Source: CAD feature listing. Evaluate the final solid. Frame: model axes, mm. A direction names the side the tool comes from. Coordinates: 2 decimals unless noted, no trailing zeros. Order: outer loops, then holes, each group sorted by start corner. A loop starts at its lowest first (then second) coordinate and runs counter-clockwise, first axis right, second up. Notation, with made-up numbers: (-15.5, -9) - (34.5, -9) arc R17 ccw to (34.5, 15) - close; hole circle Ø7 at (-7.5, -11). An arc over 180 degrees is marked (long way). One line per question, with ' | ' between items. Start each with the question number.
(1) Access query for faces 1 (the flat face through (80, 2, 24.613)), 2 (the flat face through (61, 1.588, 35)), 3 (the flat face through (1.588, 1, 36)), 4 (the flat face through (61, 1.588, 5)). Directions: +Z, -Z, +X, -X, +Y, -Y. A direction counts if a zero-diameter tool reaches every point of the face in a straight line with its end or side. Return the directions, or none.
(2) Section C-C (x = 39). Return the cut outline in (y, z) (1 decimal).
(3) Section A-A (y = 2.65). Count the separate pieces of the cut face and the enclosed holes in it, then the cut area to 3 significant figures.
(4) Section B-B (x = 112). Return the cut outline in (y, z) (1 decimal), then the cut area to 3 significant figures.
(5) Draft query along X for faces 5 (the flat face through (63, 0, 19)), 6 (the flat face through (123.825, 2, 16)), 7 (the flat face through (106, 2, 14.77)), 8 (the flat face through (0, 2, 16)). Return one class per face: +X half, -X half, draft (parallel to the pull), parting line (faces both ways), or undercut.
(6) Contact query for flat-ended pins moving along their axis: P1, Ø1, axis at y = 2.5, z = 18, coming from the -X side; P2, Ø1.6, axis at y = 2, z = 35.5, coming from the -X side; P3, Ø1, axis at y = 1.5, z = 35, coming from the +X side. Output: stop coordinate, or through.
(7) Line query: line 1 along Z through (x, y) = (106.5, 3.05) (1 decimal); line 2 along Z through (x, y) = (43.5, 1.9) (1 decimal); line 3 along X through (y, z) = (0.8, 15) (1 decimal). Output: solid intervals per line, ascending.
Autodesk Inventor part; units mm, degrees
ref_plane "YZ Plane" through (0, 0, 0) normal (1, 0, 0) x (0, 1, 0)
ref_plane "XZ Plane" through (0, 0, 0) normal (0, 1, 0) x (-1, 0, 0)
ref_plane "XY Plane" through (0, 0, 0) normal (0, 0, 1) x (1, 0, 0)
sketch "Sketch1" plane through (0, 0, 0) normal (0, 1, 0) x (-1, 0, 0)
  line L0 (0, 0) -> (-123.825, 0)
  line L1 (-123.825, 0) -> (-123.825, 38.1)
  line L2 (-123.825, 38.1) -> (0, 38.1)
  line L3 (0, 38.1) -> (0, 0)
  dimension "d0" = 123.825
  dimension "d1" = 38.1
extrude "Extrusion1" add sketch "Sketch1" along normal blind 3.175
sketch "Sketch2" plane through (0, 3.175, 0) normal (0, 1, 0) x (1, 0, 0)
  line L0 (123.825, 0) -> (0, 0)
  line L1 (0, 0) -> (0, -38.1)
  line L2 (0, -38.1) -> (123.825, -38.1)
  line L3 (123.825, -38.1) -> (123.825, 0)
  line L4 (0, -36.5125) -> (123.825, -36.5125)
  line L5 (123.825, -36.5125) -> (123.825, -33.3121)
  line L6 (123.825, -33.3121) -> (0, -33.3121)
  line L7 (0, -33.3121) -> (0, -36.5125)
  line L8 (1.5875, -3.175) -> (122.2375, -3.175)
  line L9 (122.2375, -3.175) -> (122.2375, -6.604)
  line L10 (122.2375, -6.604) -> (1.5875, -6.604)
  line L11 (1.5875, -6.604) -> (1.5875, -3.175)
  dimension "d6" = 3.2004
  dimension "d7" = 1.5875
  dimension "d10" = 3.175
  dimension "d11" = 3.429
  dimension "d12" = 1.5875
  dimension "d13" = 1.5875
extrude "Extrusion2" cut sketch "Sketch2" against normal blind 1.5875 contours L3 L4 L1 L6
sketch "Sketch3" plane through (0, 3.175, 0) normal (0, 1, 0) x (1, 0, 0)
  line L0 (123.825, -33.3121) -> (123.825, 0)
  line L1 (123.825, 0) -> (0, 0)
  line L2 (0, 0) -> (0, -33.3121)
  line L3 (1.5875, -3.175) -> (122.2375, -3.175)
  line L4 (122.2375, -3.175) -> (122.2375, -6.604)
  line L5 (122.2375, -6.604) -> (1.5875, -6.604)
  line L6 (1.5875, -6.604) -> (1.5875, -3.175)
  dimension "d14" = 1.5875
  dimension "d15" = 1.5875
  dimension "d16" = 3.175
  dimension "d17" = 3.429
extrude "Extrusion3" cut sketch "Sketch3" against normal blind 1.5875
sketch "Sketch4" plane through (0, 3.175, 0) normal (0, 1, 0) x (1, 0, 0)
  line L0 (0, -38.1) -> (1.5875, -38.1)
  line L1 (1.5875, -38.1) -> (1.5875, -31.75)
  line L2 (1.5875, -31.75) -> (0, -31.75)
  line L3 (0, -31.75) -> (0, -38.1)
  line L4 (123.825, -38.1) -> (122.2375, -38.1)
  line L5 (122.2375, -38.1) -> (122.2375, -31.75)
  line L6 (122.2375, -31.75) -> (123.825, -31.75)
  line L7 (123.825, -31.75) -> (123.825, -38.1)
  point P0 (0, 0)
  dimension "d20" = 1.5875
  dimension "d21" = 6.35
  dimension "d22" = 6.35
  dimension "d23" = 1.5875
extrude "Extrusion4" cut sketch "Sketch4" against normal blind 25.4
fillet "Fillet1" radius 1.5875 1 edges at (122.2375, 1.5875, 31.75)
fillet "Fillet2" radius 1.5875 1 edges at (1.5875, 1.5875, 31.75)
sketch "Sketch5" plane through (0, 3.175, 0) normal (0, 1, 0) x (1, 0, 0)
  line L0 (1.5873, -33.3121) -> (122.2377, -33.3121)
  line L1 (74.9935, -21.0566) -> (84.1375, -21.0566)
  line L2 (84.1375, -21.0566) -> (84.1375, -24.6126)
  line L3 (84.1375, -24.6126) -> (74.9935, -24.6126)
  line L4 (74.9935, -24.6126) -> (74.9935, -21.0566)
  line L5 (122.2375, -36.5125) -> (122.2375, -33.3375)
  dimension "d28" = 8.6995
  dimension "d29" = 3.556
  dimension "d30" = 9.144
  dimension "d44" = 38.1
extrude "Extrusion5" cut sketch "Sketch5" against normal blind 25.4
fillet "Fillet3" radius 1.5875 4 edges at (74.9935, 1.5875, 21.0566) (84.1375, 1.5875, 21.0566) (84.1375, 1.5875, 24.6126) (74.9935, 1.5875, 24.6126)
sketch "Sketch6" plane through (0, 3.175, 0) normal (0, 1, 0) x (1, 0, 0)
  line L0 (1.5873, -33.3121) -> (122.2377, -33.3121)
  line L1 (93.6625, -14.7701) -> (119.6975, -14.7701)
  line L2 (119.6975, -14.7701) -> (119.6975, -26.2001)
  line L3 (119.6975, -26.2001) -> (93.6625, -26.2001)
  line L4 (93.6625, -26.2001) -> (93.6625, -14.7701)
  line L5 (122.2375, -36.5125) -> (122.2375, -33.3375)
  dimension "d35" = 26.035
  dimension "d36" = 11.43
  dimension "d41" = 7.112
  dimension "d43" = 2.54
extrude "Extrusion6" cut sketch "Sketch6" against normal blind 25.4
properties part number "Electronics Container Part 4"
Response values:
1) face 1: +Y, -Y | face 2: +X, -X, +Y | face 3: +Z, -X, +Y, -Y | face 4: +Y
2) outline: (0, 0) - (3.2, 0) - (3.2, 3.2) - (1.6, 3.2) - (1.6, 6.6) - (3.2, 6.6) - (3.2, 33.3) - (1.6, 33.3) - (1.6, 36.5) - (3.2, 36.5) - (3.2, 38.1) - (0, 38.1) - close
3) separate pieces: 2 | enclosed holes: 3 | area: 3,570 mm²
4) outline: (0, 0) - (3.2, 0) - (3.2, 3.2) - (1.6, 3.2) - (1.6, 6.6) - (3.2, 6.6) - (3.2, 14.8) - (0, 14.8) - close; (0, 26.2) - (3.2, 26.2) - (3.2, 33.3) - (1.6, 33.3) - (1.6, 36.5) - (3.2, 36.5) - (3.2, 38.1) - (0, 38.1) - close | area: 74.2 mm²
5) face 5: draft | face 6: +X half | face 7: undercut | face 8: -X half
6) P1: stops at x = 0 | P2: stops at x = 1.59 | P3: stops at x = 122.24
7) line 1: z = 0 to 3.2, 6.6 to 14.8, 26.2 to 33.3, 36.5 to 38.1 | line 2: z = 0 to 3.2, 6.6 to 33.3, 36.5 to 38.1 | line 3: x = 0 to 93.7, 119.7 to 123.8
